Geometry: final body of the model. Coordinates: model frame, mm. Face numbers are marked on the shaded views. A direction names the side the tool comes from. Give positions to 0.01 mm unless a question says otherwise; leave off trailing zeros. Write each loop counter-clockwise with the first axis right and the second up, starting at its lowest first coordinate (ties: lowest second). Pieces come first, ordered by that corner, then holes. Notation, with made-up numbers: (61.5, -38) -> (77.5, -38) arc R24 ccw to (77.5, -1) -> close; hole circle Ø4 at (17.5, 11.25). An arc over 180 degrees is marked (long way). Answer as a JSON object with one key per item and string values. Group by question number.
(1) Section query B-B on z = -3.25. Output: boundary loops of the cut face in (x, y).
(2) Set-up query: the marked faces 4 and 5. Return all of +Z, -Z, +X, -X, +Y, -Y with unobstructed straight access to the full face (end or side cutting, diameter ignored); none if empty.
(3) Section query A-A on z = -17.25. Output: boundary loops of the cut face in (x, y), plus the area to 3 significant figures.
(4) Contact query for flat-ended pins moving along their axis: pin 1 Ø3 at (x, z) = (-0.5, -0.5) entering from +Y; pin 2 Ø1.5 at (x, z) = (0.5, -13.5) entering from +Y; pin 3 Ø1.4 at (x, z) = (0, -1) entering from -Y. Output: stop coordinate, or through.
(5) Material intervals for probe 1 along Z at (x, y) = (-5, -1.5); probe 2 along X at (y, z) = (0, -14.75); probe 3 along X at (y, z) = (-2, -1.75), sorted ascending.
(6) Draft query along Y for the marked faces 1, 2 and 3. Return one class per face: +Y half, -Y half, draft (parallel to the pull), parting line (faces both ways), or undercut.
Solid Edge part; units mm, degrees
sketch "Sketch1" plane through (0, 0, 0) normal (1, 0, 0) x (0, 1, 0)
  line L0 (0, -2.1082) -> (0, 2.1082)
  arc A0 (0, 2.1082) -> (6.9469, -2.1082) centre (-0.3606, -6.3169) cw
  line L1 (0, -2.1082) -> (6.9469, -2.1082)
revolve "RevolvedProtrusion1" add sketch "Sketch1" angle 360 about axis through (0, 0, -14.7796) along (0, 0, 1)
sketch "Sketch2" plane through (0, 0, -2.1082) normal (0, 0, -1) x (0, 1, 0)
  circle A0 centre (0, 0) radius 3.9687
extrude "Protrusion1" add sketch "Sketch2" along normal blind 19.05
sketch "Sketch3" plane through (0, 0, -21.1582) normal (0, 0, -1) x (1, 0, 0)
  circle A0 centre (0, 0) radius 3.9662
extrude "Cutout1" cut sketch "Sketch3" against normal blind 17.4625 flip side to cut
sketch "Sketch4" plane through (-0.6032, 0.3606, 4.2164) normal (0, 0, 1) x (1, 0, 0)
  line L0 (-0.7716, 2.0206) -> (1.978, 2.0206)
  line L1 (3.3529, -0.3606) -> (1.978, 2.0206)
  line L2 (1.978, -2.7419) -> (3.3529, -0.3606)
  line L3 (-0.7716, -2.7419) -> (1.978, -2.7419)
  line L4 (-2.1464, -0.3606) -> (-0.7716, -2.7419)
  line L5 (-0.7716, 2.0206) -> (-2.1464, -0.3606)
extrude "ExtrudedCutout_11" cut sketch "Sketch4" against normal blind 6.3246
properties part number "117718"
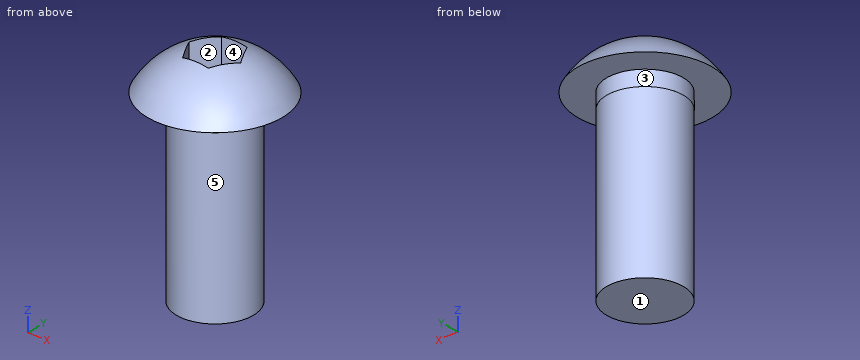
Answer list:
{
 "1": {"outline": "circle Ø7.94 at (0, 0)"},
 "2": {"face 4": "+Z", "face 5": "-Z"},
 "3": {"outline": "circle Ø7.93 at (0, 0)", "area": "49.4 mm2"},
 "4": {"pin 1": "y = 6.87", "pin 2": "y = 3.97", "pin 3": "y = -6.7"},
 "5": {"probe 1": "-2.11 to 0.01", "probe 2": "-3.97 to 3.97", "probe 3": "-6.42 to -1.59, 1.59 to 6.42"},
 "6": {"face 1": "draft", "face 2": "undercut", "face 3": "parting line"}
}
